```python
from build123d import *

# Parameters (mm, degrees)
SKETCH_1_W           = 49.5
SKETCH_1_H           = 24.5
EXTRUDE_1_DEPTH      = 36
SKETCH_2_R           = 2.5
CUT_EXTRUDE_1_DEPTH  = 3
SKETCH_3_W           = 15.4
SKETCH_3_H           = 2.7
CUT_EXTRUDE_2_DEPTH  = 12
SKETCH_9_W           = 23
SKETCH_9_H           = 49.5
CUT_EXTRUDE_9_DEPTH  = 24.5
SKETCH_11_W          = 14.5
SKETCH_11_H          = 1.9
CUT_EXTRUDE_8_DEPTH  = 2
FILLET_1_R           = 3
EXTRUDE_START        = 32.5
EXTRUDE_2_DEPTH      = 32.5
SKETCH_13_W          = 23.5
SKETCH_13_H          = 13.5
CUT_EXTRUDE_10_DEPTH = 7.6
SKETCH_14_W          = 33
SKETCH_14_H          = 13.5
CUT_EXTRUDE_11_DEPTH = 9.4
SKETCH_16_R          = 1.45
CUT_EXTRUDE_12_DEPTH = 17
SKETCH_17_R          = 3.125
CUT_EXTRUDE_13_DEPTH = 9.4
CUT_EXTRUDE_14_DEPTH = 3
CUT_EXTRUDE_START    = -49.5
CUT_EXTRUDE_15_DEPTH = 49.5
SKETCH_20_W          = 7
SKETCH_20_H          = 2.5
CUT_EXTRUDE_16_DEPTH = 19


with BuildPart() as part:
    # Эскиз1 → Бобышка-Вытянуть1 (new body)
    with BuildSketch(Plane(origin=(0, 0, 0), x_dir=(0, 0, -1), z_dir=(1, 0, 0))):
        Rectangle(SKETCH_1_W, SKETCH_1_H)
    extrude(amount=EXTRUDE_1_DEPTH)

    # Эскиз2 → Вырез-Вытянуть1 (cut)
    with BuildSketch(Plane.ZY):
        with Locations((-20, -7.25)):
            Circle(SKETCH_2_R)
        with Locations((20, -7.25)):
            Circle(SKETCH_2_R)
    extrude(amount=-CUT_EXTRUDE_1_DEPTH, mode=Mode.SUBTRACT)

    # Эскиз3 → Вырез-Вытянуть2 (cut)
    with BuildSketch(Plane.ZY):
        with Locations((0, 4.75)):
            Rectangle(SKETCH_3_W, SKETCH_3_H)
        with Locations((0, 8.75)):
            Rectangle(SKETCH_3_W, SKETCH_3_H)
    extrude(amount=-CUT_EXTRUDE_2_DEPTH, mode=Mode.SUBTRACT)

    # Эскиз9 → Вырез-Вытянуть9 (cut)
    with BuildSketch(Plane.XZ.offset(-12.25)):
        with Locations((24.5, 0)):
            Rectangle(SKETCH_9_W, SKETCH_9_H)
    extrude(amount=CUT_EXTRUDE_9_DEPTH, mode=Mode.SUBTRACT)

    # Эскиз11 → Вырез-Вытянуть8 (cut)
    with BuildSketch(Plane.ZY.offset(-12)):
        with Locations((0, 8.75)):
            Rectangle(SKETCH_11_W, SKETCH_11_H)
        with Locations((0, 4.75)):
            Rectangle(SKETCH_11_W, SKETCH_11_H)
    extrude(amount=-CUT_EXTRUDE_8_DEPTH, mode=Mode.SUBTRACT)

    # Скругление1
    fillet_1_edges = [part.edges().sort_by_distance(p)[0] for p in [
        (6.5, 12.25, -24.75),
        (6.5, -12.25, -24.75),
        (6.5, -12.25, 24.75),
        (6.5, 12.25, 24.75),
    ]]
    fillet(fillet_1_edges, radius=FILLET_1_R)

    # Эскиз12 → Бобышка-Вытянуть2 (add)
    with BuildSketch(Plane(origin=(13, 0, 0), x_dir=(0, 0, -1), z_dir=(1, 0, 0)).offset(EXTRUDE_START)):
        with BuildLine():
            Line((-7.75, 12.25), (-7.75, -12.25))
            Line((-7.75, -12.25), (-21.75, -12.25))
            ThreePointArc((-21.75, -12.25), (-23.871320344, -11.371320344), (-24.75, -9.25))
            Line((-24.75, -9.25), (-24.75, 9.25))
            ThreePointArc((-24.75, 9.25), (-23.871320344, 11.371320344), (-21.75, 12.25))
            Line((-21.75, 12.25), (-7.75, 12.25))
        make_face()
        with BuildLine():
            Line((21.75, 12.25), (7.75, 12.25))
            Line((7.75, 12.25), (7.75, -12.25))
            Line((7.75, -12.25), (21.75, -12.25))
            ThreePointArc((21.75, -12.25), (23.871320344, -11.371320344), (24.75, -9.25))
            Line((24.75, -9.25), (24.75, 9.25))
            ThreePointArc((24.75, 9.25), (23.871320344, 11.371320344), (21.75, 12.25))
        make_face()
    extrude(amount=-EXTRUDE_2_DEPTH)

    # Эскиз13 → Вырез-Вытянуть10 (cut)
    with BuildSketch(Plane(origin=(0, 0, 7.75), x_dir=(-1, 0, 0), z_dir=(0, 0, -1))):
        with Locations((-24.25, 0)):
            Rectangle(SKETCH_13_W, SKETCH_13_H)
    extrude(amount=-CUT_EXTRUDE_10_DEPTH, mode=Mode.SUBTRACT)

    # Эскиз14 → Вырез-Вытянуть11 (cut)
    with BuildSketch(Plane(origin=(0, 0, 15.35), x_dir=(-1, 0, 0), z_dir=(0, 0, -1))):
        with Locations((-24.5, 0)):
            Rectangle(SKETCH_14_W, SKETCH_14_H)
    extrude(amount=-CUT_EXTRUDE_11_DEPTH, mode=Mode.SUBTRACT)

    # Эскиз16 → Вырез-Вытянуть12 (cut)
    with BuildSketch(Plane.XY.offset(24.75)):
        with Locations((9.5, 0)):
            Circle(SKETCH_16_R)
        with Locations((39, 0)):
            Circle(SKETCH_16_R)
    extrude(amount=-CUT_EXTRUDE_12_DEPTH, mode=Mode.SUBTRACT)

    # Эскиз17 → Вырез-Вытянуть13 (cut)
    with BuildSketch(Plane.XY.offset(24.75)):
        with Locations((9.5, 0)):
            Circle(SKETCH_17_R)
        with Locations((39, 0)):
            Circle(SKETCH_17_R)
    extrude(amount=-CUT_EXTRUDE_13_DEPTH, mode=Mode.SUBTRACT)

    # Эскиз18 → Вырез-Вытянуть14 (cut)
    with BuildSketch(Plane.XY.offset(-7.75)):
        with BuildLine():
            Line((31.875, 2.875), (45.5, 2.875))
            Line((45.5, 2.875), (45.5, -3.125))
            Line((45.5, -3.125), (31.875, -3.125))
            ThreePointArc((31.875, -3.125), (28.875, -0.125), (31.875, 2.875))
        make_face()
    extrude(amount=-CUT_EXTRUDE_14_DEPTH, mode=Mode.SUBTRACT)

    # Эскиз19 → Вырез-Вытянуть15 (cut)
    with BuildSketch(Plane(origin=(0, 0, -24.75), x_dir=(-1, 0, 0), z_dir=(0, 0, -1)).offset(CUT_EXTRUDE_START)):
        with BuildLine():
            Line((-33.25, 12.25), (-46.5, 12.25))
            Line((-46.5, 12.25), (-46.5, -12.25))
            Line((-46.5, -12.25), (-33.25, -12.25))
            ThreePointArc((-33.25, -12.25), (-45.5, 0), (-33.25, 12.25))
        make_face()
    extrude(amount=CUT_EXTRUDE_15_DEPTH, mode=Mode.SUBTRACT)

    # Эскиз20 → Вырез-Вытянуть16 (cut)
    with BuildSketch(Plane.XY.offset(24.75)):
        with Locations((20, 9.5)):
            Rectangle(SKETCH_20_W, SKETCH_20_H)
    extrude(amount=-CUT_EXTRUDE_16_DEPTH, mode=Mode.SUBTRACT)


solid = part.part
```
Check sheet for the modelled part. Datum: model origin and axes. Units: mm. A direction names the side the tool comes from. Coordinates: 2 decimals unless noted, no trailing zeros. Write each loop counter-clockwise with the first axis right and the second up, starting at its lowest first coordinate (ties: lowest second). Pieces come first, ordered by that corner, then holes. Notation, with made-up numbers: (-19, 46.25) - (0, 46.25) arc R13 ccw to (0, 66.25) - close; hole circle Ø4 at (13, -14). An arc over 180 degrees is marked (long way). One line per question, with ' | ' between items.
Item 1: Sectioned sample at C-C on z = 1.5. Record the boundary of the cut face in (x, y).
Determined:
outline: (0, -12.25) - (13, -12.25) - (13, 3.8) - (12, 3.8) - (12, 3.4) - (0, 3.4) - close; (0, 6.1) - (12, 6.1) - (12, 5.7) - (13, 5.7) - (13, 7.8) - (12, 7.8) - (12, 7.4) - (0, 7.4) - close; (0, 10.1) - (12, 10.1) - (12, 9.7) - (13, 9.7) - (13, 12.25) - (0, 12.25) - close
Item 2: Mould release check, pull along Z, two halves, no side actions. Record for faces 6 (the face through (10, 2, 15.35)), 7 (the face through (8, 5, 20)), 8 (the face through (6, 3.4, 0)): pulls with the +Z half, pulls with the -Z half, needs draft (parallel to the pull), parting line crosses it, or undercut.
Determined:
face 6: pulls with the +Z half | face 7: needs draft | face 8: undercut
Item 3: Sectioned sample at A-A on z = -20. Record the boundary of the cut face in (x, y).
Determined:
outline: (0, -12.25) - (33.25, -12.25) arc R12.25 ccw to (33.25, 12.25) - (0, 12.25) - (0, -4.75) - (3, -4.75) - (3, -9.75) - (0, -9.75) - close
Item 4: Thickness scan on line 1 (Z direction, x = 7.5, y = 8.25); line 2 (Z direction, x = 29.5, y = -8.25); line 3 (Y direction, x = 1, z = -20). Record the ranges inside material, lowest first. Write a range as [from, to].
Determined:
line 1: z = [-24.75, -7.7], [7.7, 24.75] | line 2: z = [-24.75, -7.75], [7.75, 24.75] | line 3: y = [-12.25, -9.75], [-4.75, 12.25]
Item 5: Sectioned sample at B-B on x = 9.5. Record the boundary of the cut face in (y, z), plus the area to 3 significant figures.
Determined:
outline: (-12.25, -21.75) arc R3 ccw to (-9.25, -24.75) - (9.25, -24.75) arc R3 ccw to (12.25, -21.75) - (12.25, 21.75) arc R3 ccw to (9.25, 24.75) - (6.75, 24.75) - (6.75, 15.35) - (1.45, 15.35) - (1.45, 7.75) - (-1.45, 7.75) - (-1.45, 15.35) - (-6.75, 15.35) - (-6.75, 24.75) - (-9.25, 24.75) arc R3 ccw to (-12.25, 21.75) - close; hole (3.4, -7.7) - (6.1, -7.7) - (6.1, 7.7) - (3.4, 7.7) - close; hole (7.4, -7.7) - (10.1, -7.7) - (10.1, 7.7) - (7.4, 7.7) - close | area: 973 mm2
Item 6: Access from +Z, -Z, +X, -X, +Y, -Y to the whole of each face (thin tool, end or side, straight path). Record for faces 1 (the face through (8.05, 0.06, 11.6)), 2 (the face through (28.876, -0.191, -9.229)), 3 (the face through (6, 5, -7.7)), 4 (the face through (26, 0, -7.75)), 5 (the face through (37, 0, -10.75)).
Determined:
face 1: +Z | face 2: +Z, +X | face 3: -X | face 4: +X, +Y, -Y | face 5: +X
Item 7: Gauge pin test, flat ends, axial feed: P1, Ø2, axis at x = 12.5, y = 3, coming from the +Z side; P2, Ø3, axis at y = 9, z = 19.5, coming from the +X side; P3, Ø1.8, axis at x = 10, y = 0, coming from the +Z side. Record the tip position at first contact, or that the pin passes through.
Determined:
P1: stops at z = 15.35 | P2: stops at x = 42.94 | P3: stops at z = 7.75
Item 8: Sectioned sample at D-D on x = 15. Record the boundary of the cut face in (y, z), plus the area to 3 significant figures.
Determined:
outline: (-12.25, -21.75) arc R3 ccw to (-9.25, -24.75) - (9.25, -24.75) arc R3 ccw to (12.25, -21.75) - (12.25, -7.75) - (-12.25, -7.75) - close; (-12.25, 7.75) - (-6.75, 7.75) - (-6.75, 24.75) - (-9.25, 24.75) arc R3 ccw to (-12.25, 21.75) - close; (6.75, 7.75) - (12.25, 7.75) - (12.25, 21.75) arc R3 ccw to (9.25, 24.75) - (6.75, 24.75) - close | area: 596 mm2
